Input: part model. Units: mm. Frame: model coordinates. Coordinates: 2 decimals unless noted, no trailing zeros. Loops run counter-clockwise (first coordinate to the right, second up) from the corner with the lowest first, then second, coordinate; pieces in that order, holes last.
(1) Contact query for flat-ended pins moving along their axis: P1, Ø6.5, axis at x = 99.5, y = -43.5, coming from the -Z side; P2, Ø4, axis at y = 31, z = -15.5, coming from the +X side. Output: stop coordinate, or through.
(2) Section A-A, the plane x = 105. Return loops of the section in (y, z), then the cut area to 3 significant figures.
(3) Line query: L1, parallel to Y at x = 0, z = 8.25; L2, parallel to X at y = 0, z = 10.75; L3, parallel to Y at x = 140, z = -43. Output: solid intervals per line, ascending.
(4) Section C-C, the plane z = -122.5. Return loops of the section in (x, y).
(5) Section D-D, the plane z = 2.5. Return loops of the section in (x, y).
(6) Section B-B, the plane y = 0. Return loops of the section in (x, z).
```python
from build123d import *

# Parameters (mm, degrees)
F1_DEPTH = 15
F3_DEPTH = 160


# Not quite as in the source:
# - after a boolean that leaves OpenCascade's solid faulty, fix() repairs it


with BuildPart() as f1:
    # F0 (on Top) → F1 (new body)
    with BuildSketch(Plane.XY):
        with BuildLine():
            ThreePointArc((41.3226906327, -22.3927496943), (52.5, -15.7816452182), (63.6773093673, -22.3927496943))
            ThreePointArc((63.6773093673, -22.3927496943), (63.7058777697, -22.4450182881), (63.7342017495, -22.4974197353))
            ThreePointArc((63.7342017494, -22.4974197352), (152, 0), (63.7342017494, 22.4974197352))
            ThreePointArc((63.7342017494, 22.4974197352), (63.7058777696, 22.445018288), (63.6773093673, 22.3927496943))
            ThreePointArc((63.6773093673, 22.3927496943), (52.5, 15.7816452182), (41.3226906327, 22.3927496943))
            ThreePointArc((41.3226906327, 22.3927496943), (41.2941222304, 22.445018288), (41.2657982506, 22.4974197352))
            ThreePointArc((41.2657982506, 22.4974197352), (-47, 0), (41.2657982506, -22.4974197352))
            ThreePointArc((41.2657982506, -22.4974197352), (41.2941222304, -22.445018288), (41.3226906327, -22.3927496943))
        make_face()
        with BuildLine():
            ThreePointArc((39.5041211148, 21.5505084615), (39.5355894457, 21.4927235868), (39.5669732516, 21.4348927618))
            ThreePointArc((39.5669732516, 21.4348927618), (52.5, 13.7816452182), (65.4330267484, 21.4348927618))
            ThreePointArc((65.4330267484, 21.4348927618), (65.4644105543, 21.4927235868), (65.4958788852, 21.5505084615))
            ThreePointArc((65.4958788852, 21.5505084615), (150, 0), (65.4958788852, -21.5505084615))
            ThreePointArc((65.4958788852, -21.5505084615), (65.4644105543, -21.4927235868), (65.4330267484, -21.4348927618))
            ThreePointArc((65.4330267484, -21.4348927618), (63.4899302841, -18.6916573179), (60.976304449, -16.4594723499))
            ThreePointArc((60.976304449, -16.4594723499), (49.1601952928, -14.1646192224), (39.5669732516, -21.4348927618))
            ThreePointArc((39.5669732516, -21.4348927618), (39.5355894457, -21.4927235868), (39.5041211148, -21.5505084615))
            ThreePointArc((39.5041211148, -21.5505084615), (-45, 0), (39.5041211148, 21.5505084615))
        make_face(mode=Mode.SUBTRACT)
    extrude(amount=F1_DEPTH)

    # F2 (on face) → F3 (join)
    with BuildSketch(Plane(origin=(0, 0, 0), x_dir=(1, 0, 0), z_dir=(0, 0, -1))):
        with BuildLine():
            ThreePointArc((74.7889823447, 36.0040888266), (73.2472602421, 34.6520348301), (71.7659812842, 33.2340187158))
            Line((71.7659812842, 33.2340187158), (73.1801948457, 31.8198051543))
            ThreePointArc((73.1801948466, 31.8198051534), (74.5984406573, 33.1774801565), (76.0745575641, 34.4719999404))
            Line((76.0745575641, 34.4719999404), (74.7889823447, 36.0040888266))
        make_face()
        with BuildLine():
            ThreePointArc((71.7659812842, 33.2340187158), (70.3479651699, 31.7527397579), (68.9959111734, 30.2110176553))
            Line((68.9959111734, 30.2110176553), (70.5280000596, 28.9254424359))
            ThreePointArc((70.5280000596, 28.9254424359), (71.8225198435, 30.4015593427), (73.1801948466, 31.8198051534))
            Line((73.1801948457, 31.8198051543), (71.7659812842, 33.2340187158))
        make_face()
        with BuildLine():
            ThreePointArc((141.0040888266, 30.2110176553), (138.2340187158, 33.2340187158), (135.2110176553, 36.0040888266))
            Line((135.2110176553, 36.0040888266), (133.9254424359, 34.4719999404))
            ThreePointArc((133.9254424359, 34.4719999404), (136.8198051534, 31.8198051534), (139.4719999404, 28.9254424359))
            Line((139.4719999404, 28.9254424359), (141.0040888266, 30.2110176553))
        make_face()
        with BuildLine():
            ThreePointArc((135.2110176553, -36.0040888266), (138.2340187158, -33.2340187158), (141.0040888266, -30.2110176553))
            Line((141.0040888266, -30.2110176553), (139.4719999404, -28.9254424359))
            ThreePointArc((139.4719999404, -28.9254424359), (136.8198051534, -31.8198051534), (133.9254424359, -34.4719999404))
            Line((133.9254424359, -34.4719999404), (135.2110176553, -36.0040888266))
        make_face()
        with BuildLine():
            Line((70.5280000596, -28.9254424359), (68.9959111734, -30.2110176553))
            ThreePointArc((68.9959111734, -30.2110176553), (71.7659812842, -33.2340187158), (74.7889823447, -36.0040888266))
            Line((74.7889823447, -36.0040888266), (76.0745575641, -34.4719999404))
            ThreePointArc((76.0745575641, -34.4719999404), (73.1801948466, -31.8198051534), (70.5280000596, -28.9254424359))
        make_face()
    extrude(amount=F3_DEPTH)

    add(f1.part.fix(), mode=Mode.REPLACE)


solid = f1.part
```
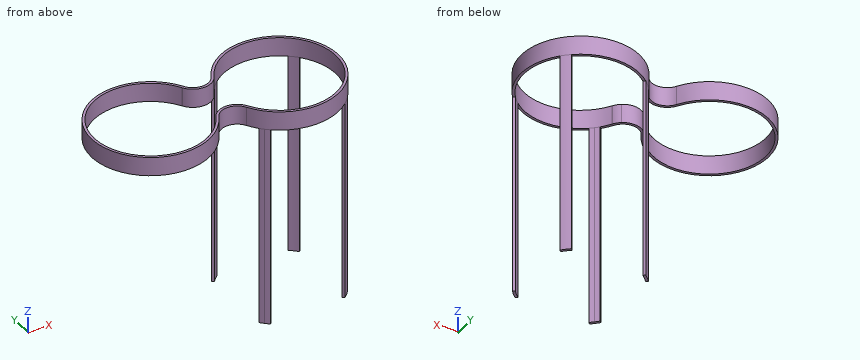
Report:
1. P1: stops at z = 0
1. P2: stops at x = 141
2. outline: (-47, 0) - (-45, 0) - (-45, 15) - (-47, 15) - close; (45, 0) - (47, 0) - (47, 15) - (45, 15) - close
2. area: 60.0 mm2
3. L1: y = -47 to -45, 45 to 47
3. L2: x = -47 to -45, 150 to 152
3. L3: y = -31.37 to -29.37, 29.37 to 31.37
4. outline: (69, -30.21) arc R47 ccw to (74.79, -36) - (76.07, -34.47) arc R45 cw to (70.53, -28.93) - close; (69, 30.21) - (70.53, 28.93) arc R45 cw to (76.07, 34.47) - (74.79, 36) arc R47 ccw to start; (133.93, -34.47) - (135.21, -36) arc R47 ccw to (141, -30.21) - (139.47, -28.93) arc R45 cw to start; (133.93, 34.47) arc R45 cw to (139.47, 28.93) - (141, 30.21) arc R47 ccw to (135.21, 36) - close
5. outline: (41.27, -22.5) arc R12.75 cw to (41.32, -22.39) arc R12.75 cw to (63.73, -22.5) arc R47 ccw (long way) to (63.73, 22.5) arc R12.75 cw to (63.68, 22.39) arc R12.75 cw to (41.32, 22.39) arc R12.75 cw to (41.27, 22.5) arc R47 ccw (long way) to start; hole (39.5, -21.55) arc R45 ccw to (39.57, -21.43) arc R14.75 cw to (65.43, -21.43) arc R45 ccw to (65.5, -21.55) arc R45 ccw (long way) to (65.5, 21.55) arc R45 ccw to (65.43, 21.43) arc R14.75 cw to (39.57, 21.43) arc R45 ccw to (39.5, 21.55) arc R45 ccw (long way) to start
6. outline: (-47, 0) - (-45, 0) - (-45, 15) - (-47, 15) - close; (150, 0) - (152, 0) - (152, 15) - (150, 15) - close
